```python
from build123d import *

# Parameters (mm, degrees)
SKETCH1_R           = 1
CASING_DEPTH        = 16.2
CASING_CHAMFER_SIZE = 0.1
SKETCH3_R           = 0.35
SKETCH4_R           = 0.25
EXPOSED_WIRE_DEPTH  = 0.5


with BuildPart() as part:
    # Sketch1 → Casing (new body)
    with BuildSketch(Plane.XY):
        Circle(SKETCH1_R)
    extrude(amount=CASING_DEPTH)

    # Casing Chamfer
    casing_chamfer_edges = [part.edges().sort_by_distance(p)[0] for p in [
        (-1, 0, 0),
        (-1, 0, 16.2),
    ]]
    chamfer(casing_chamfer_edges, length=CASING_CHAMFER_SIZE)

    # Wire 2: sweep along a path in Sketch2
    with BuildLine(Plane(origin=(0, 0, 0), x_dir=(1, 0, 0), z_dir=(0, 1, 0))) as wire_2_path:
        Line((0, 0), (0, 1.2))
        ThreePointArc((0, 1.2), (0.234314575, 1.765685425), (0.8, 2))
        Line((0.8, 2), (30.5, 2))
    # Sketch3 → Wire 2 (sweep)
    with BuildSketch(Plane(origin=(0, 0, 0), x_dir=(-1, 0, 0), z_dir=(0, 0, -1))):
        with Locations((0, -0.4)):
            Circle(SKETCH3_R)
        with Locations((0, 0.4)):
            Circle(SKETCH3_R)
    sweep(path=wire_2_path.line)

    # Sketch4 → Exposed Wire (add)
    with BuildSketch(Plane(origin=(30.5, 0, 0), x_dir=(0, 0, -1), z_dir=(1, 0, 0))):
        with Locations((2, 0.4)):
            Circle(SKETCH4_R)
        with Locations((2, -0.4)):
            Circle(SKETCH4_R)
    extrude(amount=EXPOSED_WIRE_DEPTH)


solid = part.part
```
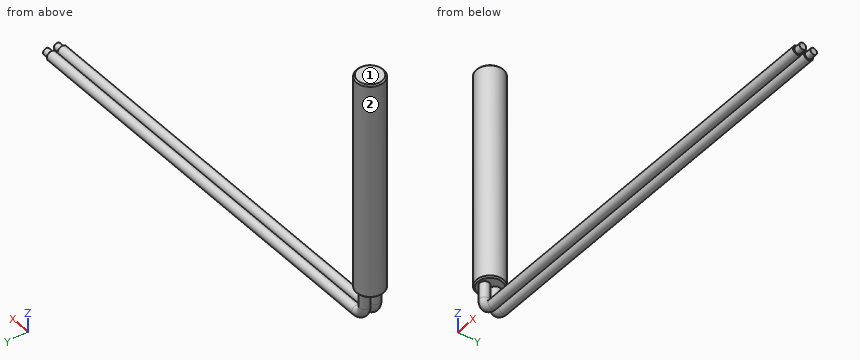
For this review, take the finished solid that the model builds, in its own axes (mm). Face numbers are marked on the shaded views. A direction names the side the tool comes from. Round coordinates to 2 decimals unless told otherwise and drop trailing zeros. Write each loop counter-clockwise with the first axis right and the second up, starting at its lowest first coordinate (ties: lowest second). Pieces come first, ordered by that corner, then holes. Notation, with made-up numbers: (68.25, -32.5) -> (73.25, -32.5) arc R28 cw to (73.25, 3.5) -> close; hole circle Ø11 at (-15.5, 65). An arc over 180 degrees is marked (long way). One line per question, with ' | ' between items. Start each with the question number.
(1) Add section A-A, the plane x = 22. Write out the cut boundary in (y, z), plus the area to 3 significant figures.
(2) Tool access review of the marked faces 1 and 2: name each direction out of +Z, -Z, +X, -X, +Y, -Y from which nothing blocks a thin tool from reaching the whole face with its end or side.
(3) For line 1 along Z through (x, y) = (11.5, 0.45); line 2 along X through (y, z) = (-0.05, 2.5); line 3 along Z through (x, y) = (6, 0.65), list the stretches that pass through material, from the lowest coordinate up. Write a range as from..to.
(4) Insertion check: P1, Ø0.5, axis at x = 0.5, y = 0, coming from the -Z side; P2, Ø6, axis at x = 8, z = 0, coming from the +Y side. Each pin has a flat end and moves straight along its axis. Give the tip position at first contact, or say it passes through.
(5) Add section B-B, the plane z = 5.5. Write out the cut boundary in (x, y).
Answer list:
1) outline: circle Ø0.7 at (-0.4, -2); circle Ø0.7 at (0.4, -2) | area: 0.770 mm²
2) face 1: +Z, +X, -X, +Y, -Y | face 2: +Z
3) line 1: -2.35..-1.65 | line 2: -1..1 | line 3: -2.24..-1.76
4) P1: z = -2.29 | P2: y = 0.75
5) outline: circle Ø2 at (0, 0)
